Part model, mm, in its own coordinate system. Face numbers are marked on the shaded views. A direction names the side the tool comes from. Give positions to 0.01 mm unless a question says otherwise; leave off trailing zeros. Order: outer loops, then holes, each group sorted by start corner. A loop starts at its lowest first (then second) coordinate and runs counter-clockwise, first axis right, second up. Notation, with made-up numbers: (68, 4.25) -> (82, 4.25) arc R7 ccw to (82, 14.25) -> close; hole circle Ø6 at (28, -18). An arc over 180 degrees is marked (long way). Write item = value, one per line. Start each with the question number.
Item 1: Band-saw the part on A-A on z = 15.5. Write the cut outline in (x, y).
Item 2: Band-saw the part on B-B on x = 14.5. Write the cut outline in (y, z), plus the area to 3 significant figures.
Item 3: Tool access for the marked faces 1 and 2: list every direction of +Z, -Z, +X, -X, +Y, -Y with a clear straight run to the whole face (end or side of a thin tool).
Item 4: Band-saw the part on C-C on y = 14. Write the cut outline in (x, z), plus the area to 3 significant figures.
Item 5: Flat gauge pins, fed straight in: P1, Ø1.5, axis at x = -37, y = 44.5, coming from the +Z side; P2, Ø1.5, axis at x = -36.5, y = 43.5, coming from the +Z side; P3, Ø3, axis at x = 48.5, y = -25, coming from the +Z side. Where does each tip first touch, or does it go through?
Item 6: Band-saw the part on D-D on x = 36. Write the cut outline in (y, z), plus the area to 3 significant figures.
Item 7: Drill centre lines: line 1 along Y through (x, z) = (36, 4.35); line 2 along Y through (x, z) = (31.5, 17.25); line 3 along X through (y, z) = (-39, 5). Where is each one in solid material? Low to high.
Item 8: Pull direction Y, two halves, no side cores. Call the marked faces 3, 4 and 5: +Y half, -Y half, draft (parallel to the pull), parting line (faces both ways), or undercut.
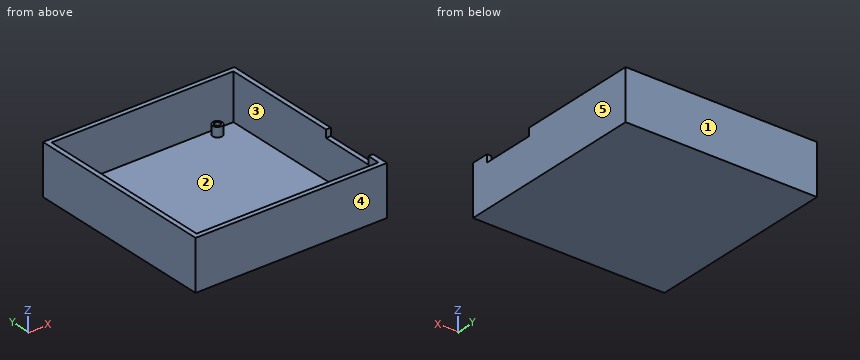
Autodesk Inventor part; units mm, degrees
ref_plane "YZ Plane" through (0, 0, 0) normal (1, 0, 0) x (0, 1, 0)
ref_plane "XZ Plane" through (0, 0, 0) normal (0, 1, 0) x (-1, 0, 0)
ref_plane "XY Plane" through (0, 0, 0) normal (0, 0, 1) x (1, 0, 0)
sketch "Esboço1" plane through (0, 0, 0) normal (0, 0, 1) x (1, 0, 0)
  line L0 (-50, 50.5) -> (50, 50.5)
  line L1 (50, 50.5) -> (50, -50.5)
  line L2 (50, -50.5) -> (-50, -50.5)
  line L3 (-50, -50.5) -> (-50, 50.5)
  line L4 (-50, 50.5) -> (50, -50.5) construction
  line L5 (50, 50.5) -> (-50, -50.5) construction
  point P0 (0, 0)
  dimension "d0" = 100
  dimension "d1" = 101
extrude "Base" add sketch "Esboço1" along normal blind 26
sketch "Esboço2" plane through (0, 0, 26) normal (0, 0, 1) x (1, 0, 0)
  line L0 (50, 50.5) -> (-50, 50.5)
  line L1 (-50, -50.5) -> (50, -50.5)
  line L2 (-50, 50.5) -> (50, 50.5)
  line L3 (50, 50.5) -> (50, -50.5)
  line L4 (50, -50.5) -> (-50, -50.5)
  line L5 (-50, -50.5) -> (-50, 50.5)
  line L6 (47.5, -48) -> (47.5, 48)
  line L7 (47.5, 48) -> (-47.5, 48)
  line L8 (-47.5, 48) -> (-47.5, -48)
  line L9 (-47.5, -48) -> (47.5, -48)
  point P0 (0, 0)
  dimension "d4" = 2.5
extrude "Área" cut sketch "Esboço2" against normal blind 24 contours L9 L8 L7 L6
sketch "Esboço3" plane through (0, 0, 2) normal (0, 0, 1) x (1, 0, 0)
  circle A0 centre (-36, -44) radius 1.5
  line L0 (-50, 50.5) -> (-50, -50.5)
  line L1 (-50, -50.5) -> (50, -50.5)
  line L2 (-47.5, -48) -> (-47.5, 48)
  line L3 (47.5, 48) -> (47.5, -48)
  circle A1 centre (-36, 44) radius 1.5
  circle A2 centre (36, -44) radius 1.5
  circle A3 centre (36, 44) radius 1.5
  circle A4 centre (-36, -44) radius 2.5
  line L4 (47.5, -48) -> (-47.5, -48)
  line L5 (-47.5, 48) -> (47.5, 48)
  circle A5 centre (-36, 44) radius 2.5
  circle A6 centre (36, -44) radius 2.5
  circle A7 centre (36, 44) radius 2.5
  dimension "d11" = 3
  dimension "d12" = 14
  dimension "d13" = 6.5
  dimension "d14" = 5
extrude "Extrusão3" add sketch "Esboço3" along normal blind 5 contours A4 | A5 | A6 | A7
sketch "Esboço4" plane through (50, -50.5, 0) normal (1, 0, 0) x (0, 0, -1)
  line L0 (-26, 9.2) -> (-22, 9.2)
  line L1 (-22, 9.2) -> (-22, 37.2)
  line L2 (-22, 37.2) -> (-26, 37.2)
  line L3 (-26, 37.2) -> (-26, 9.2)
  point P0 (0, 50.5)
  dimension "d17" = 4
  dimension "d18" = 28
extrude "Extrusão4" cut sketch "Esboço4" against normal up to surface (2.5 mm away)
properties part number "Base ESP_3DPrint"
Values found:
q1.outline = (-50, -50.5) -> (50, -50.5) -> (50, 50.5) -> (-50, 50.5) -> close; hole (-47.5, -48) -> (47.5, -48) -> (47.5, 48) -> (-47.5, 48) -> close
q2.outline = (-50.5, 0) -> (50.5, 0) -> (50.5, 26) -> (48, 26) -> (48, 2) -> (-48, 2) -> (-48, 26) -> (-50.5, 26) -> close
q2.area = 322 mm^2
q3.face_1 = +Z, -Z, +X, -X, +Y
q3.face_2 = +Z
q4.outline = (-50, 0) -> (50, 0) -> (50, 26) -> (47.5, 26) -> (47.5, 2) -> (-47.5, 2) -> (-47.5, 26) -> (-50, 26) -> close
q4.area = 320 mm^2
q5.P1 = 7
q5.P2 = 2
q5.P3 = 22
q6.outline = (-50.5, 0) -> (50.5, 0) -> (50.5, 26) -> (48, 26) -> (48, 2) -> (46.5, 2) -> (46.5, 7) -> (45.5, 7) -> (45.5, 2) -> (42.5, 2) -> (42.5, 7) -> (41.5, 7) -> (41.5, 2) -> (-41.5, 2) -> (-41.5, 7) -> (-42.5, 7) -> (-42.5, 2) -> (-45.5, 2) -> (-45.5, 7) -> (-46.5, 7) -> (-46.5, 2) -> (-48, 2) -> (-48, 26) -> (-50.5, 26) -> close
q6.area = 342 mm^2
q7.line_1 = -50.5 to -48, -46.5 to -45.5, -42.5 to -41.5, 41.5 to 42.5, 45.5 to 46.5, 48 to 50.5
q7.line_2 = -50.5 to -48, 48 to 50.5
q7.line_3 = -50 to -47.5, 47.5 to 50
q8.face_3 = undercut
q8.face_4 = -Y half
q8.face_5 = draft
